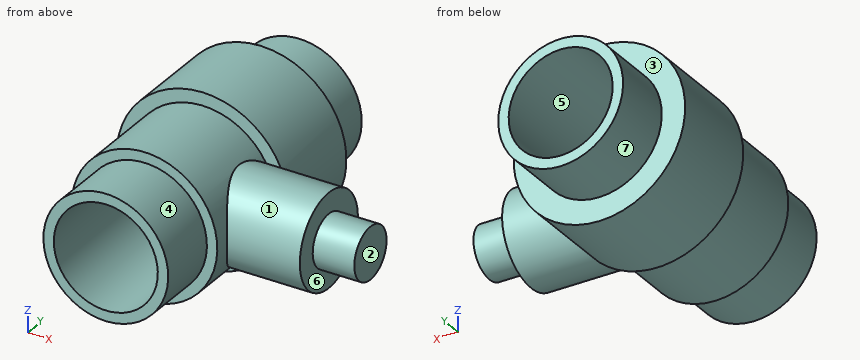
```python
from build123d import *

# Parameters (mm, degrees)
SKETCH1_R                = 10.4775
BOSS_EXTRUDE1_DEPTH      = 11.43
SKETCH2_R                = 8.89
BOSS_EXTRUDE2_DEPTH      = 11.43
BOSS_EXTRUDE3_DEPTH      = 7.62
BOSS_EXTRUDE3_DEPTH_BACK = 30.48
SKETCH3_R                = 7.62
SKETCH4_R                = 5.715
BOSS_EXTRUDE4_DEPTH      = 17.78
SKETCH5_R                = 3.175
BOSS_EXTRUDE5_DEPTH      = 5.08
SKETCH6_R                = 6.35
CUT_EXTRUDE1_DEPTH       = 46.650494065


with BuildPart() as part:
    # Sketch1 → Boss-Extrude1 (new body)
    with BuildSketch(Plane(origin=(0, 0, 0), x_dir=(1, 0, 0), z_dir=(0, 1, 0))):
        with Locations(Location((0, 0, 0), (0, 0, 270))):
            Circle(SKETCH1_R)
    extrude(amount=BOSS_EXTRUDE1_DEPTH)

    # Sketch2 → Boss-Extrude2 (add)
    with BuildSketch(Plane.XZ):
        with Locations(Location((0, 0, 0), (0, 0, 270))):
            Circle(SKETCH2_R)
    extrude(amount=BOSS_EXTRUDE2_DEPTH)

    # Sketch3 → Boss-Extrude3 (add, two sides: drawn at the far end of the back side and taken through both)
    with BuildSketch(Plane.XZ.offset(11.43).offset(-BOSS_EXTRUDE3_DEPTH_BACK)):
        with Locations(Location((0, 0, 0), (0, 0, 270))):
            Circle(SKETCH3_R)
    extrude(amount=BOSS_EXTRUDE3_DEPTH + BOSS_EXTRUDE3_DEPTH_BACK)

    # Sketch4 → Boss-Extrude4 (add)
    with BuildSketch(Plane(origin=(0, 0, 0), x_dir=(0, 0, -1), z_dir=(1, 0, 0))):
        with Locations(Location((0, -3.81, 0), (0, 0, 221.810313572))):
            Circle(SKETCH4_R)
    extrude(amount=BOSS_EXTRUDE4_DEPTH)

    # Sketch5 → Boss-Extrude5 (add)
    with BuildSketch(Plane(origin=(17.78, 0, 0), x_dir=(0, 0, -1), z_dir=(1, 0, 0))):
        with Locations((0, -3.81)):
            Circle(SKETCH5_R)
    extrude(amount=BOSS_EXTRUDE5_DEPTH)

    # Sketch6 → Cut-Extrude1 (cut, through all)
    with BuildSketch(Plane(origin=(0, 19.05, 0), x_dir=(1, 0, 0), z_dir=(0, 1, 0))):
        with Locations(Location((0, 0, 0), (0, 0, 270))):
            Circle(SKETCH6_R)
    extrude(amount=-CUT_EXTRUDE1_DEPTH, mode=Mode.SUBTRACT)


solid = part.part
```
The model under review builds one solid part; all positions refer to its coordinate system, in mm. Face numbers are marked on the shaded views. A direction names the side the tool comes from. Round coordinates to 2 decimals unless told otherwise and drop trailing zeros. Write each loop counter-clockwise with the first axis right and the second up, starting at its lowest first coordinate (ties: lowest second). Pieces come first, ordered by that corner, then holes. Notation, with made-up numbers: (68, 58) - (102, 58) arc R19 ccw to (102, 84) - close; hole circle Ø2 at (10.25, -7.75). An arc over 180 degrees is marked (long way). Use one line per item in the form item = value.
Q1. Consider section C-C (y = -3.81). State the section outline as (x, z) points (3 decimals), and give its area (3 significant figures).
Answer key:
outline = (6.81, -5.715) - (17.78, -5.715) - (17.78, -3.175) - (22.86, -3.175) - (22.86, 3.175) - (17.78, 3.175) - (17.78, 5.715) - (6.81, 5.715) arc R8.89 ccw (long way) to start; hole circle Ø12.7 at (0, 0)
area = 263 mm2
Q2. Consider section D-D (z = -2.5). State the section outline as (x, y) points.
Answer key:
outline = (-10.17, 0) - (-8.53, 0) - (-8.53, -11.43) - (-7.2, -11.43) - (-7.2, -19.05) - (-5.84, -19.05) - (-5.84, 19.05) - (-7.2, 19.05) - (-7.2, 11.43) - (-10.17, 11.43) - close; (5.84, -19.05) - (7.2, -19.05) - (7.2, -11.43) - (8.53, -11.43) - (8.53, -8.95) - (17.78, -8.95) - (17.78, -5.77) - (22.86, -5.77) - (22.86, -1.85) - (17.78, -1.85) - (17.78, 1.33) - (10.17, 1.33) - (10.17, 11.43) - (7.2, 11.43) - (7.2, 19.05) - (5.84, 19.05) - close
Q3. Consider section B-B (x = 0). State the section outline as (y, z) points, and give its area (3 significant figures).
Answer key:
outline = (-19.05, -7.62) - (-11.43, -7.62) - (-11.43, -8.89) - (0, -8.89) - (0, -10.48) - (11.43, -10.48) - (11.43, -7.62) - (19.05, -7.62) - (19.05, -6.35) - (-19.05, -6.35) - close; (-19.05, 6.35) - (19.05, 6.35) - (19.05, 7.62) - (11.43, 7.62) - (11.43, 10.48) - (0, 10.48) - (0, 8.89) - (-11.43, 8.89) - (-11.43, 7.62) - (-19.05, 7.62) - close
area = 191 mm2
Q4. Draft analysis for pull direction Z (two halves, no side actions). For the marked faces 5, 6 and 7, state which applies: +Z half, -Z half, draft (parallel to the pull), parting line (faces both ways), or undercut.
Answer key:
face_5 = undercut
face_6 = draft
face_7 = parting line
Q5. For line 1 (X direction, y = -10, z = 0); line 2 (X direction, y = 8, z = 0); line 3 (Y direction, x = 4, z = -7), list the stretches that pass through material, from the lowest coordinate up. Write a range as [from, to].
Answer key:
line_1 = [-8.89, -6.35], [6.35, 8.89]
line_2 = [-10.48, -6.35], [6.35, 10.48]
line_3 = [-11.43, 11.43]
Q6. Tool access review of the marked faces 1, 2, 3 and 4: name each direction out of +Z, -Z, +X, -X, +Y, -Y from which nothing blocks a thin tool from reaching the whole face with its end or side.
Answer key:
face_1 = +X
face_2 = +Z, -Z, +X, +Y, -Y
face_3 = +Y
face_4 = -Y
Q7. Insertion check: pin 1 Ø1 at (x, y) = (18, -8) entering from +Z; pin 2 Ø1.5 at (y, z) = (-8, -1) entering from +X; pin 3 Ø1 at (x, y) = (13.5, -1.5) entering from -Z. Each pin has a flat end and moves straight along its axis. Give the tip position at first contact, or say it passes through.
Answer key:
pin_1 = 4.32
pin_2 = 17.78
pin_3 = -5.42
